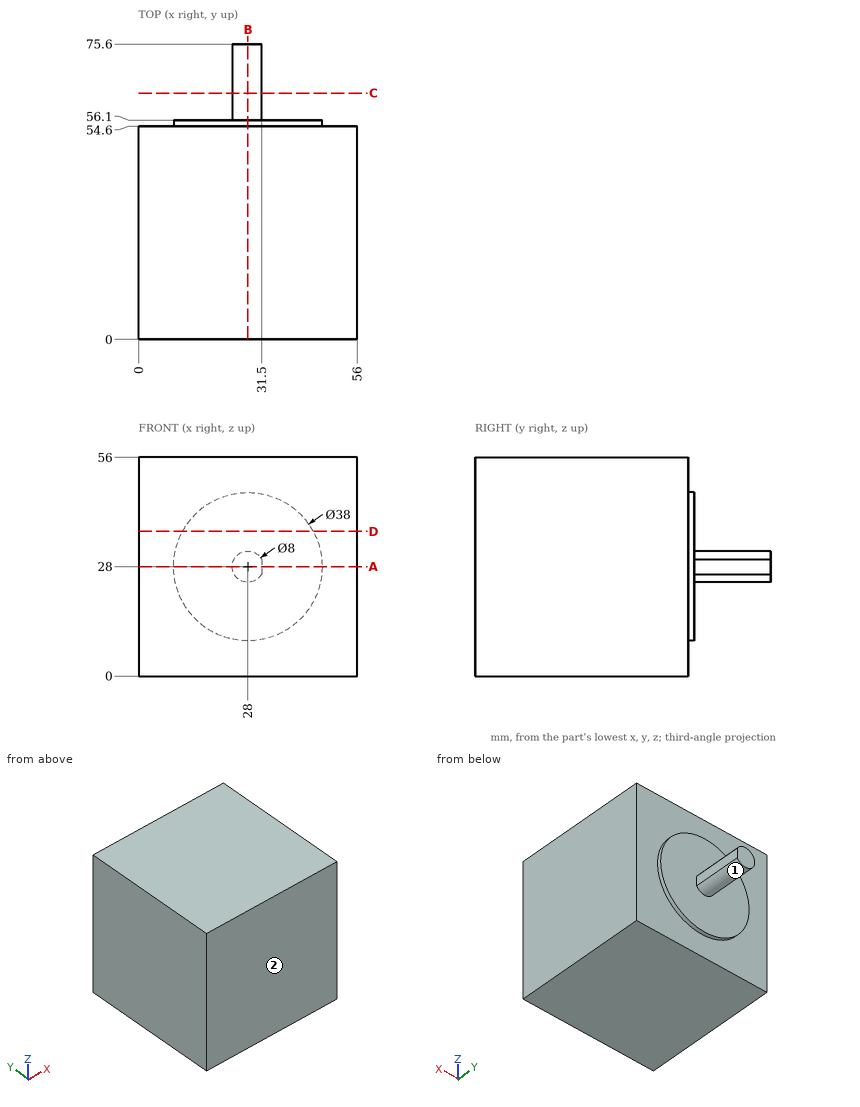
Here's the drawing with two shaded views (mm, measured from the low corner). I have some questions. A direction names the side the tool comes from. Coordinates: 2 decimals unless noted, no trailing zeros. Loops run counter-clockwise (first coordinate to the right, second up) from the corner with the lowest first, then second, coordinate; pieces in that order, holes last. Notation, with made-up numbers: M -32.75,30 L 15.25,30 A21 ccw 15.25,43 Z; hole C 54.5,-25.75 d4. An arc over 180 degrees is marked long. Put each result on its own line as item: value. Start each with the question number.
(1) I need wall thicknesses on probe 1 along Y at (x, z) = (8, 22); probe 2 along Y at (x, z) = (32, 16); probe 3 along Z at (x, y) = (43, 55). Which ranges of each line are inside material? Lowest first, please.
(2) Imagine slicing it at A-A on z = 28. List the corners of the cut face in (x, y) for me.
(3) Which directions (+Z, -Z, +X, -X, +Y, -Y) give clear straight access to the entire face, cutting with the end or side of a thin tool? Please do the marked faces 1 and 2.
(4) Imagine slicing it at B-B on x = 28. List the corners of the cut face in (y, z) for me, and give its area (3 significant figures).
(5) Will these pins go through, and if not, where does the flat tip stop? pin 1 Ø4.5 at (y, z) = (61.5, 28) entering from +X; pin 2 Ø2 at (x, z) = (19, 16.5) entering from +Y; pin 3 Ø6 at (x, z) = (43, 11) entering from +Y.
(6) Imagine slicing it at C-C on y = 63. List the corners of the cut face in (x, z) for me, and give its area (3 significant figures).
(7) Imagine slicing it at D-D on z = 37. List the corners of the cut face in (x, y) for me, and give its area (3 significant figures).
Worked answers:
1. probe 1: y = 0 to 54.6
1. probe 2: y = 0 to 56.1
1. probe 3: z = 16.34 to 39.66
2. outline: M 0,0 L 56,0 L 56,54.6 L 47,54.6 L 47,56.1 L 31.5,56.1 L 31.5,75.6 L 24,75.6 L 24,56.1 L 9,56.1 L 9,54.6 L 0,54.6 Z
3. face 1: +Y
3. face 2: +Z, -Z, +X, -X, -Y
4. outline: M 0,0 L 54.6,0 L 54.6,9 L 56.1,9 L 56.1,24 L 75.6,24 L 75.6,32 L 56.1,32 L 56.1,47 L 54.6,47 L 54.6,56 L 0,56 Z
4. area: 3,270 mm2
5. pin 1: stops at x = 31.5
5. pin 2: stops at y = 56.1
5. pin 3: stops at y = 54.6
6. outline: M 31.5,26.06 L 31.5,29.94 A4 ccw long Z
6. area: 49.0 mm2
7. outline: M 0,0 L 56,0 L 56,54.6 L 44.73,54.6 L 44.73,56.1 L 11.27,56.1 L 11.27,54.6 L 0,54.6 Z
7. area: 3,110 mm2
